Geometry: final body of the model. Coordinates: model frame, mm. A direction names the side the tool comes from. Round coordinates to 2 decimals unless told otherwise and drop trailing zeros. Order: outer loops, then holes, each group sorted by start corner. A loop starts at its lowest first (then second) coordinate and runs counter-clockwise, first axis right, second up. Notation, with made-up numbers: (62, -2.75) - (73, -2.75) arc R38 cw to (73, 35.25) - close; hole circle Ø2 at (45, 51.5). An arc over 180 degrees is marked (long way). Put each result on its own line as item: value. Start each with the question number.
(1) Pin query (flat end, axial travel): P1, Ø1.5, axis at y = 7.5, z = 4.5, coming from the +X side; P2, Ø1.5, axis at y = -6, z = 6, coming from the -X side; P3, Ø1, axis at y = -2.5, z = 1, coming from the -X side. Return the tip coordinate at first contact, or that it passes through.
(2) Section D-D (x = -18). Output: boundary loops of the cut face in (y, z), and give its area (3 significant figures).
(3) Section B-B (y = 0.75). Output: boundary loops of the cut face in (x, z).
(4) Pull-direction query (Y, two-part tool) for faces 4 (the face through (0, 10, 8)), 5 (the face through (-15.04, -1.05, 3.17)), 6 (the face through (0, 0, 10)); classes: released by +Y, released by -Y, zero draft, split by the parting line, or undercut.
(5) Material intervals for L1, parallel to Y at x = 12.5, z = 2.5; L2, parallel to Y at x = -12.5, z = 8.5; L3, parallel to Z at x = 14, y = 4.5, sorted ascending. Write a range as [from, to].
(6) Section A-A (z = 3). Count the separate pieces of the cut face and the enclosed holes in it, and give its area (3 significant figures).
(7) Access query for faces 1 (the face through (19.65, 6.99, 5.07)), 2 (the face through (-4, 0, 2)), 3 (the face through (-18.614, 0.269, 8.235)). Directions: +Z, -Z, +X, -X, +Y, -Y. A direction counts if a zero-diameter tool reaches every point of the face in a straight line with its end or side. Return the directions, or none.
(8) Section C-C (x = -11). Output: boundary loops of the cut face in (y, z).
from build123d import *

# Parameters (mm, degrees)
SKETCH2_W                               = 45
SKETCH2_H                               = 20
BOSS_EXTRUDE2_DEPTH                     = 10
FILLET1_R                               = 10
CUT_EXTRUDE1_DEPTH                      = 22
CBORE_FOR_M5_HEX_HEAD_BOLT1_D           = 5.5
CBORE_FOR_M5_HEX_HEAD_BOLT1_CBORE_D     = 12.24
CBORE_FOR_M5_HEX_HEAD_BOLT1_CBORE_DEPTH = 3.58


with BuildPart() as part:
    # Sketch2 → Boss-Extrude2 (new body)
    with BuildSketch(Plane.XY):
        Rectangle(SKETCH2_W, SKETCH2_H)
    extrude(amount=BOSS_EXTRUDE2_DEPTH)

    # Fillet1
    fillet1_edges = [part.edges().sort_by_distance(p)[0] for p in [
        (22.5, 10, 5),
        (22.5, -10, 5),
        (-22.5, 10, 5),
        (-22.5, -10, 5),
    ]]
    fillet(fillet1_edges, radius=FILLET1_R - 0.0001)  # a hair under: the kernel refuses the full size

    # Sketch3 → Cut-Extrude1 (cut)
    with BuildSketch(Plane.XZ.offset(10)):
        with BuildLine():
            Line((-4, 0), (-4, 3.5))
            ThreePointArc((-4, 3.5), (0, 7.5), (4, 3.5))
            Line((4, 3.5), (4, 0))
            ThreePointArc((4, 0), (0, -4), (-4, 0))
        make_face()
    extrude(amount=-CUT_EXTRUDE1_DEPTH, mode=Mode.SUBTRACT)

    # CBORE for M5 Hex Head Bolt1 (through all)
    with Locations(Plane.XY.offset(10)):
        with Locations((-12.5, 0), (12.5, 0)):
            CounterBoreHole(CBORE_FOR_M5_HEX_HEAD_BOLT1_D / 2, CBORE_FOR_M5_HEX_HEAD_BOLT1_CBORE_D / 2, CBORE_FOR_M5_HEX_HEAD_BOLT1_CBORE_DEPTH)


solid = part.part
Checks:
1. P1: stops at x = 19.88
1. P2: stops at x = -21.01
1. P3: stops at x = -22.3
2. outline: (-8.35, 0) - (8.35, 0) - (8.35, 10) - (2.68, 10) - (2.68, 6.42) - (-2.68, 6.42) - (-2.68, 10) - (-8.35, 10) - close
2. area: 148 mm²
3. outline: (-22.47, 0) - (-15.15, 0) - (-15.15, 6.42) - (-18.57, 6.42) - (-18.57, 10) - (-22.47, 10) - close; (-9.85, 0) - (-4, 0) - (-4, 3.5) arc R4 cw to (4, 3.5) - (4, 0) - (9.85, 0) - (9.85, 6.42) - (6.43, 6.42) - (6.43, 10) - (-6.43, 10) - (-6.43, 6.42) - (-9.85, 6.42) - close; (15.15, 0) - (22.47, 0) - (22.47, 10) - (18.57, 10) - (18.57, 6.42) - (15.15, 6.42) - close
4. face 4: released by +Y
4. face 5: undercut
4. face 6: zero draft
5. L1: y = [-10, -2.75], [2.75, 10]
5. L2: y = [-10, -6.12], [6.12, 10]
5. L3: z = [0, 6.42]
6. separate pieces: 2
6. enclosed holes: 2
6. area: 607 mm²
7. face 1: +Z, -Z, +X, +Y
7. face 2: -Z, +Y, -Y
7. face 3: +Z
8. outline: (-10, 0) - (-2.3, 0) - (-2.3, 6.42) - (-5.93, 6.42) - (-5.93, 10) - (-10, 10) - close; (2.3, 0) - (10, 0) - (10, 10) - (5.93, 10) - (5.93, 6.42) - (2.3, 6.42) - close
